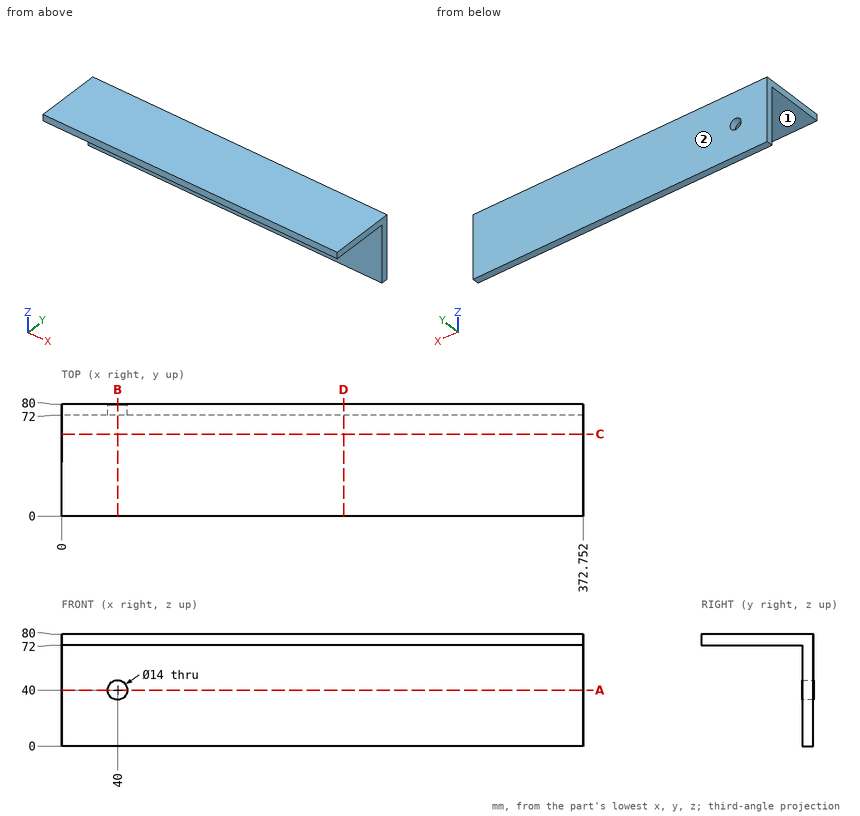
Geometry check sheet. Reference: drawing and pictorial views, mm from the part's lowest x, y, z. A direction names the side the tool comes from. Round coordinates to 2 decimals unless told otherwise and drop trailing zeros. Write each loop counter-clockwise with the first axis right and the second up, starting at its lowest first coordinate (ties: lowest second). Pieces come first, ordered by that corner, then holes.
1. Section check C-C on y = 58.5. Enter the section's corners in (x, z), plus the area to 3 significant figures.
2. Section check A-A on z = 40. Enter the section's corners in (x, y).
3. Scan lines: L1, parallel to X at y = 74.5, z = 40; L2, parallel to Y at x = 241.5, z = 45. Record each from-to range of solid material in increasing order.
4. Access from +Z, -Z, +X, -X, +Y, -Y to the whole of each face (thin tool, end or side, straight path). Record for the marked faces 1 and 2.
5. Gauge pin test, flat ends, axial feed: P1, Ø21.5, axis at x = 216.5, y = 25, coming from the -Z side; P2, Ø8.5, axis at x = 40, z = 40, coming from the -Y side; P3, Ø21.5, axis at x = 126.5, z = 39, coming from the -Y side. Record the tip position at first contact, or that the pin passes through.
6. Section check D-D on x = 201.5. Enter the section's corners in (y, z).
7. Section check B-B on x = 40. Enter the section's corners in (y, z).
Answer:
1. outline: (0, 72) - (372.75, 72) - (372.75, 80) - (0, 80) - close
1. area: 2,980 mm2
2. outline: (0, 72) - (33, 72) - (33, 80) - (0, 80) - close; (47, 72) - (372.75, 72) - (372.75, 80) - (47, 80) - close
3. L1: x = 0 to 33, 47 to 372.75
3. L2: y = 72 to 80
4. face 1: -Z, +X, -X, -Y
4. face 2: +Z, -Z, +X, -X, +Y
5. P1: stops at z = 72
5. P2: passes through
5. P3: stops at y = 72
6. outline: (0, 72) - (72, 72) - (72, 0) - (80, 0) - (80, 80) - (0, 80) - close
7. outline: (0, 72) - (72, 72) - (72, 47) - (80, 47) - (80, 80) - (0, 80) - close; (72, 0) - (80, 0) - (80, 33) - (72, 33) - close
